Check sheet for the modelled part. Datum: model origin and axes. Units: mm. Face numbers are marked on the shaded views. A direction names the side the tool comes from. Coordinates: 2 decimals unless noted, no trailing zeros. Loops run counter-clockwise (first coordinate to the right, second up) from the corner with the lowest first, then second, coordinate; pieces in that order, holes last. Notation, with made-up numbers: M 49.25,61 L 55.25,61 A36 ccw 55.25,96 Z; hole C 12.5,48 d2. An arc over 180 degrees is marked long. Use CSV: the item, a comma, the result in double quotes. Start each with the question number.
(1) Set-up check for the marked faces 1 and 2: record each of +Z, -Z, +X, -X, +Y, -Y from which the full face is reachable in a straight line by a thin tool's end or side.
(2) Section check D-D on z = 5. Record the cut outline in (x, y).
(3) Go/stop test with flat-tipped pins: pin 1 Ø5.5 at (x, y) = (-18, 0) entering from +Z; pin 2 Ø1.8 at (x, y) = (-26.25, -1) entering from +Z; pin 3 Ø1.5 at (x, z) = (-26, 4) entering from -Y. Record where each tip stops, or that it passes through.
(4) Section check C-C on x = 12.5. Record the cut outline in (y, z), and give its area (3 significant figures).
(5) Scan lines: line 1 (Y direction, x = 26.25, z = 1.4); line 2 (Z direction, x = -32, y = 3.5); line 3 (Z direction, x = 23, y = -0.75). Record each from-to range of solid material in increasing order.
(6) Section check B-B on y = -1. Record the cut outline in (x, z).
(7) Section check A-A on x = -26.25. Record the cut outline in (y, z).
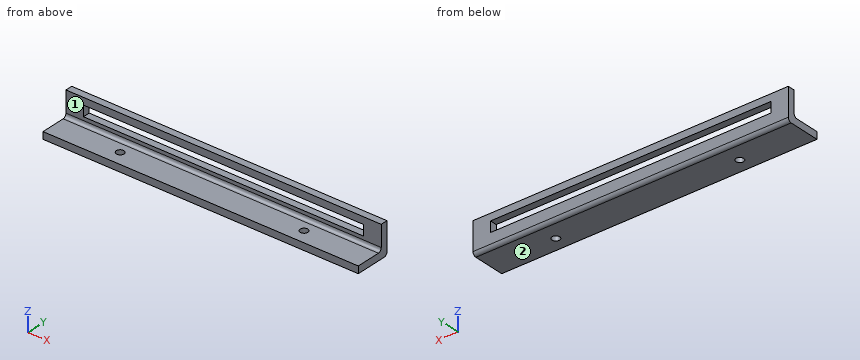
from build123d import *

# Parameters (mm, degrees)
F0_W     = 90
F0_H     = 10
F0_R     = 1.1
F1_DEPTH = 2
F2_W     = 90
F2_H     = 2
F3_DEPTH = 7
F4_R     = 1
F5_W     = 80
F5_H     = 3
F6_DEPTH = 2


with BuildPart() as f1:
    # F0 (on Top) → F1 (new body)
    with BuildSketch(Plane.XY):
        Rectangle(F0_W, F0_H)
        with Locations((-26.25, -1)):
            Circle(F0_R, mode=Mode.SUBTRACT)
        with Locations((26.25, -1)):
            Circle(F0_R, mode=Mode.SUBTRACT)
    extrude(amount=F1_DEPTH)

    # F2 (on face) → F3 (join)
    with BuildSketch(Plane.XY.offset(2)):
        with Locations((0, 4)):
            Rectangle(F2_W, F2_H)
    extrude(amount=F3_DEPTH)

    # F4
    f4_edges = [f1.edges().sort_by_distance(p)[0] for p in [
        (0, 5, 0),
        (0, 3, 2),
    ]]
    fillet(f4_edges, radius=F4_R)

    # F5 (on face) → F6 (cut)
    with BuildSketch(Plane.XZ.offset(-3)):
        with Locations((0, 5.5)):
            Rectangle(F5_W, F5_H)
    extrude(amount=-F6_DEPTH, mode=Mode.SUBTRACT)


solid = f1.part
Outcome:
1,face 1,"+Z, +X, -X, -Y"
1,face 2,"-Z, +X, -X, +Y, -Y"
2,outline,"M -45,3 L -40,3 L -40,5 L -45,5 Z; M 40,3 L 45,3 L 45,5 L 40,5 Z"
3,pin 1,"stops at z = 2.34"
3,pin 2,"passes through"
3,pin 3,"stops at y = 3"
4,outline,"M -5,0 L 4,0 A1 ccw 5,1 L 5,4 L 3,4 L 3,3 A1 cw 2,2 L -5,2 Z; M 3,7 L 5,7 L 5,9 L 3,9 Z"
4,area,"28.0 mm²"
5,line 1,"y = -5 to -2.1, 0.1 to 5"
5,line 2,"z = 0 to 4, 7 to 9"
5,line 3,"z = 0 to 2"
6,outline,"M -45,0 L -27.35,0 L -27.35,2 L -45,2 Z; M -25.15,0 L 25.15,0 L 25.15,2 L -25.15,2 Z; M 27.35,0 L 45,0 L 45,2 L 27.35,2 Z"
7,outline,"M -5,0 L -2.1,0 L -2.1,2 L -5,2 Z; M 0.1,0 L 4,0 A1 ccw 5,1 L 5,4 L 3,4 L 3,3 A1 cw 2,2 L 0.1,2 Z; M 3,7 L 5,7 L 5,9 L 3,9 Z"
